Source: CAD feature listing. Evaluate the final solid. Frame: model axes, mm. A direction names the side the tool comes from. Round coordinates to 2 decimals unless told otherwise and drop trailing zeros. Loops run counter-clockwise (first coordinate to the right, second up) from the corner with the lowest first, then second, coordinate; pieces in that order, holes last.
Item 1: Ray query, L1, parallel to Y at x = 160, z = 6.35; L2, parallel to Y at x = -21.5, z = -11; L3, parallel to Z at x = 28, y = -48. Return the intervals inside material, ascending.
Item 2: Section query A-A on x = 14. Return loops of the section in (y, z), then the cut area to 3 significant figures.
Item 3: Access query for faces 5 (the flat face through (158, -78, 5)), 6 (the flat face through (-2, 89, -7)), 7 (the flat face through (152, 85, 10)). Directions: +Z, -Z, +X, -X, +Y, -Y. A direction counts if a zero-diameter tool reaches every point of the face in a straight line with its end or side. Return the directions, or none.
Item 4: Section query B-B on y = -23. Return loops of the section in (x, z).
Item 5: Pull-direction query (Y, two-part tool) for faces 1 (the flat face through (-2, -90, -5)), 2 (the flat face through (-2, 1, 0)), 3 (the flat face through (152, -80, 10)), 4 (the flat face through (3, 90, -5)); classes: released by +Y, released by -Y, zero draft, split by the parting line, or undercut.
Item 6: First-contact query: P1, Ø3, axis at x = 160, y = 85, coming from the +Z side; P2, Ø1.5, axis at y = 85.5, z = 7.5, coming from the -X side; P3, Ø2, axis at x = -2.5, y = -24.5, coming from the +Z side; P4, Ø1.5, axis at x = 50.5, y = -58, coming from the -Z side. Flat tips, straight axial feed; report the tip coordinate or a pass-through.
```python
from build123d import *

# Parameters (mm, degrees)
F0_W      = 310
F0_H      = 180
F1_DEPTH  = 5
F2_W      = 25
F2_H      = 10
F3_DEPTH  = 5
F5_D      = 5
F6_W      = 25
F6_H      = 10
F7_DEPTH  = 5
F9_D      = 5
F10_W     = 310
F10_H     = 1
F11_DEPTH = 15
F13_D     = 5
F15_D     = 5


with BuildPart() as f1:
    # F0 (on Top) → F1 (new body)
    with BuildSketch(Plane.XY):
        Rectangle(F0_W, F0_H)
    extrude(amount=F1_DEPTH)

    # F2 (on face) → F3 (join)
    with BuildSketch(Plane.XY.offset(5)):
        with Locations((152.5, 85)):
            Rectangle(F2_W, F2_H)
    extrude(amount=F3_DEPTH)

    # F5 (through all)
    with Locations(Plane.XY.offset(10)):
        with Locations((160, 85)):
            Hole(F5_D / 2)

    # F6 (on face) → F7 (join)
    with BuildSketch(Plane.XY.offset(5)):
        with Locations((152.5, -80)):
            Rectangle(F6_W, F6_H)
    extrude(amount=F7_DEPTH)

    # F9 (through all)
    with Locations(Plane.XY.offset(10)):
        with Locations((160, -80)):
            Hole(F9_D / 2)

    # F10 (on face) → F11 (join)
    with BuildSketch(Plane(origin=(0, 0, 0), x_dir=(1, 0, 0), z_dir=(0, 0, -1))):
        with Locations((0, -89.5)):
            Rectangle(F10_W, F10_H)
        with Locations((0, 89.5)):
            Rectangle(F10_W, F10_H)
    extrude(amount=F11_DEPTH)

    # F13 (through all)
    with Locations(Plane(origin=(0, 90, 0), x_dir=(-1, 0, 0), z_dir=(0, 1, 0))):
        with Locations((-135, -7.5)):
            Hole(F13_D / 2)

    # F15 (through all)
    with Locations(Plane(origin=(0, 90, 0), x_dir=(-1, 0, 0), z_dir=(0, 1, 0))):
        with Locations((135, -7.5)):
            Hole(F15_D / 2)


solid = f1.part
```
Data:
1. L1: y = -85 to -82.5, -77.5 to -75, 80 to 82.5, 87.5 to 90
1. L2: y = -90 to -89, 89 to 90
1. L3: z = 0 to 5
2. outline: (-90, -15) - (-89, -15) - (-89, 0) - (89, 0) - (89, -15) - (90, -15) - (90, 5) - (-90, 5) - close
2. area: 930 mm2
3. face 5: -Z, +X, +Y, -Y
3. face 6: -Z, +X, -X
3. face 7: +Z, +X, -X, +Y, -Y
4. outline: (-155, 0) - (155, 0) - (155, 5) - (-155, 5) - close
5. face 1: released by -Y
5. face 2: undercut
5. face 3: zero draft
5. face 4: released by +Y
6. P1: passes through
6. P2: stops at x = 140
6. P3: stops at z = 5
6. P4: stops at z = 0
